```python
from build123d import *

# Parameters (mm, degrees)
SKETCH1_W           = 36.83
SKETCH1_H           = 37.846
BOSS_EXTRUDE1_DEPTH = 2.54
SKETCH2_R           = 1.905
BOSS_EXTRUDE2_DEPTH = 12.7
SKETCH3_R           = 15.24
BOSS_EXTRUDE3_DEPTH = 35.56
SKETCH4_W           = 36.83
SKETCH4_H           = 3.657403599
BOSS_EXTRUDE4_DEPTH = 35.56
SKETCH5_R           = 2.032
CUT_EXTRUDE1_DEPTH  = 35.56


with BuildPart() as part:
    # Sketch1 → Boss-Extrude1 (new body)
    with BuildSketch(Plane.XY):
        Rectangle(SKETCH1_W, SKETCH1_H)
    extrude(amount=BOSS_EXTRUDE1_DEPTH)

    # Sketch2 → Boss-Extrude2 (add)
    with BuildSketch(Plane.XY.offset(2.54)):
        with Locations(Location((0, 0, 0), (0, 0, 180))):  # turned: the seam where the file's is
            Circle(SKETCH2_R)
    extrude(amount=BOSS_EXTRUDE2_DEPTH)

    # Sketch3 → Boss-Extrude3 (add)
    with BuildSketch(Plane(origin=(0, 0, 0), x_dir=(-1, 0, 0), z_dir=(0, 0, -1))):
        Circle(SKETCH3_R)
    extrude(amount=BOSS_EXTRUDE3_DEPTH)

    # Sketch4 → Boss-Extrude4 (add)
    with BuildSketch(Plane(origin=(0, 0, 0), x_dir=(-1, 0, 0), z_dir=(0, 0, -1))):
        with Locations((0, -17.094298201)):
            Rectangle(SKETCH4_W, SKETCH4_H)
    extrude(amount=BOSS_EXTRUDE4_DEPTH)

    # Sketch5 → Cut-Extrude1 (cut)
    with BuildSketch(Plane.XY.offset(2.54)):
        with Locations((13.335, 13.843)):
            Circle(SKETCH5_R)
        with Locations((-12.065, 13.843)):
            Circle(SKETCH5_R)
        with Locations((-12.065, -11.557)):
            Circle(SKETCH5_R)
        with Locations((13.335, -11.557)):
            Circle(SKETCH5_R)
    extrude(amount=-CUT_EXTRUDE1_DEPTH, mode=Mode.SUBTRACT)


solid = part.part
```
CAD build for the part. Positions are in the model's coordinates, mm. A direction names the side the tool comes from. Coordinates: 2 decimals unless noted, no trailing zeros. Order: outer loops, then holes, each group sorted by start corner. A loop starts at its lowest first (then second) coordinate and runs counter-clockwise, first axis right, second up. Notation, with made-up numbers: (77, -35) - (112, -35) arc R22 ccw to (112, -5) - close; hole circle Ø11 at (37.5, 19). An arc over 180 degrees is marked (long way). Answer in a Markdown table with one row per item.
1. Slice it at D-D, the plane y = 0. List the corners of the cut face in (x, z) (3 decimals), then the cut area to 3 significant figures.
Answer:
| item | result |
|---|---|
| outline | (-18.415, 0) - (-15.24, 0) - (-15.24, -35.56) - (15.24, -35.56) - (15.24, 0) - (18.415, 0) - (18.415, 2.54) - (1.905, 2.54) - (1.905, 15.24) - (-1.905, 15.24) - (-1.905, 2.54) - (-18.415, 2.54) - close |
| area | 1,230 mm² |
2. Pull direction X, two halves, no side cores. Call faces 4 (the face through (-10.973, 15.556, 1.288)), 5 (the face through (18.415, -16, -11)), 6 (the face through (-10.8, -10.4, -33.02)), 7 (the face through (-10.35, -10.47, -11.21)): +X half, -X half, draft (parallel to the pull), parting line (faces both ways), or undercut.
Answer:
| item | result |
|---|---|
| face 4 | undercut |
| face 5 | +X half |
| face 6 | draft |
| face 7 | undercut |
3. Slice it at A-A, the plane x = 0. List the corners of the cut face in (y, z) (3 decimals).
Answer:
| item | result |
|---|---|
| outline | (-18.923, -35.56) - (-15.266, -35.56) - (-15.266, 0) - (-15.24, 0) - (-15.24, -35.56) - (15.24, -35.56) - (15.24, 0) - (18.923, 0) - (18.923, 2.54) - (1.905, 2.54) - (1.905, 15.24) - (-1.905, 15.24) - (-1.905, 2.54) - (-18.923, 2.54) - close |
4. Slice it at B-B, the plane y = 13. List the corners of the cut face in (x, z) (3 decimals).
Answer:
| item | result |
|---|---|
| outline | (-18.415, 0) - (-13.914, 0) - (-13.914, 2.54) - (-18.415, 2.54) - close; (-10.216, 0) - (-7.953, 0) - (-7.953, -35.56) - (7.953, -35.56) - (7.953, 0) - (11.486, 0) - (11.486, 2.54) - (-10.216, 2.54) - close; (15.184, 0) - (18.415, 0) - (18.415, 2.54) - (15.184, 2.54) - close |
5. Slice it at C-C, the plane z = -18. List the corners of the cut face in (x, y) (3 decimals).
Answer:
| item | result |
|---|---|
| outline | (-18.415, -18.923) - (18.415, -18.923) - (18.415, -15.266) - (-18.415, -15.266) - close; (-11.891, -9.532) arc R2.032 cw to (-10.035, -11.47) arc R15.24 ccw (long way) to start |
6. Flat gauge pins, fed straight in: P1, Ø0.9, axis at x = -10.5, y = -10, coming from the +Z side; P2, Ø1, axis at y = -10, z = -4.5, coming from the -X side; P3, Ø6.5, axis at x = 13.335, y = 13.843, coming from the -Z side. Where does each tip first touch, or does it go through?
Answer:
| item | result |
|---|---|
| P1 | z = 2.54 |
| P2 | x = -11.92 |
| P3 | z = 0 |
7. 3-axis set-ups, long thin cutter, end or side, ignore diameter. For faces 1 (the face through (0.25, -1.89, 8.8)), 2 (the face through (0, 18.923, 1)), 3 (the face through (7.9, 13.5, 0)): which of +Z, -Z, +X, -X, +Y, -Y reach the whole face in a straight line?
Answer:
| item | result |
|---|---|
| face 1 | +Z |
| face 2 | +Z, -Z, +X, -X, +Y |
| face 3 | -Z |
8. Drill centre lines: L1, parallel to Z at x = 3, y = 8.5; L2, parallel to Z at x = -16, y = 5; L3, parallel to Y at x = -8.5, z = -11. Where is each one in solid material? Low to high. Write a range as from..to.
Answer:
| item | result |
|---|---|
| L1 | -35.56..2.54 |
| L2 | 0..2.54 |
| L3 | -18.92..-15.27, -12.65..12.65 |
